Could you check a few things on this drawing? It's one solid part, dimensions in mm from its lowest x, y, z. A direction names the side the tool comes from. Give positions to 0.01 mm unless a question says otherwise; leave off trailing zeros. Loops run counter-clockwise (first coordinate to the right, second up) from the corner with the lowest first, then second, coordinate; pieces in that order, holes last. Notation, with made-up numbers: M 72.25,55 L 97.25,55 A19 ccw 97.25,88 Z; hole C 48.5,81.5 d8. An arc over 180 degrees is marked long. Answer as CSV lines item,"result". Start each with the question number.
Item 1: Will these pins go through, and if not, where does the flat tip stop? P1, Ø12, axis at x = 9.5, z = 9, coming from the -Y side; P2, Ø4, axis at x = 17.5, z = 22, coming from the +Y side; P3, Ø1.5, axis at x = 4, y = 7, coming from the -Z side; P4, Ø4, axis at x = 2.5, z = 23.5, coming from the +Y side.
Item 2: I want a section at D-D on y = 2.5. List the corners of the cut face in (x, z) for me, plus the area to 3 significant figures.
Item 3: I want a section at A-A on z = 14. List the corners of the cut face in (x, y) for me.
Item 4: I want a section at B-B on x = 11.25. List the corners of the cut face in (y, z) for me.
Item 5: If we mould it in two halves opening along Y, with no side actions, what happens to the marked faces 3, 4 and 5? For each: released by +Y, released by -Y, zero draft, split by the parting line, or undercut.
Item 6: For the marked faces 1 and 2, which set-ups out of +Z, -Z, +X, -X, +Y, -Y let a thin tool reach every point of the face, with its end or its side?
Item 7: I want a section at C-C on y = 12.25. List the corners of the cut face in (x, z) for me.
Item 8: If I drill on line 1 along X through (y, z) = (10, 27.25); line 2 along Z through (x, y) = (10, 3.95), over which ranges is the centre line in solid material (lowest first)? Write a range as from..to.
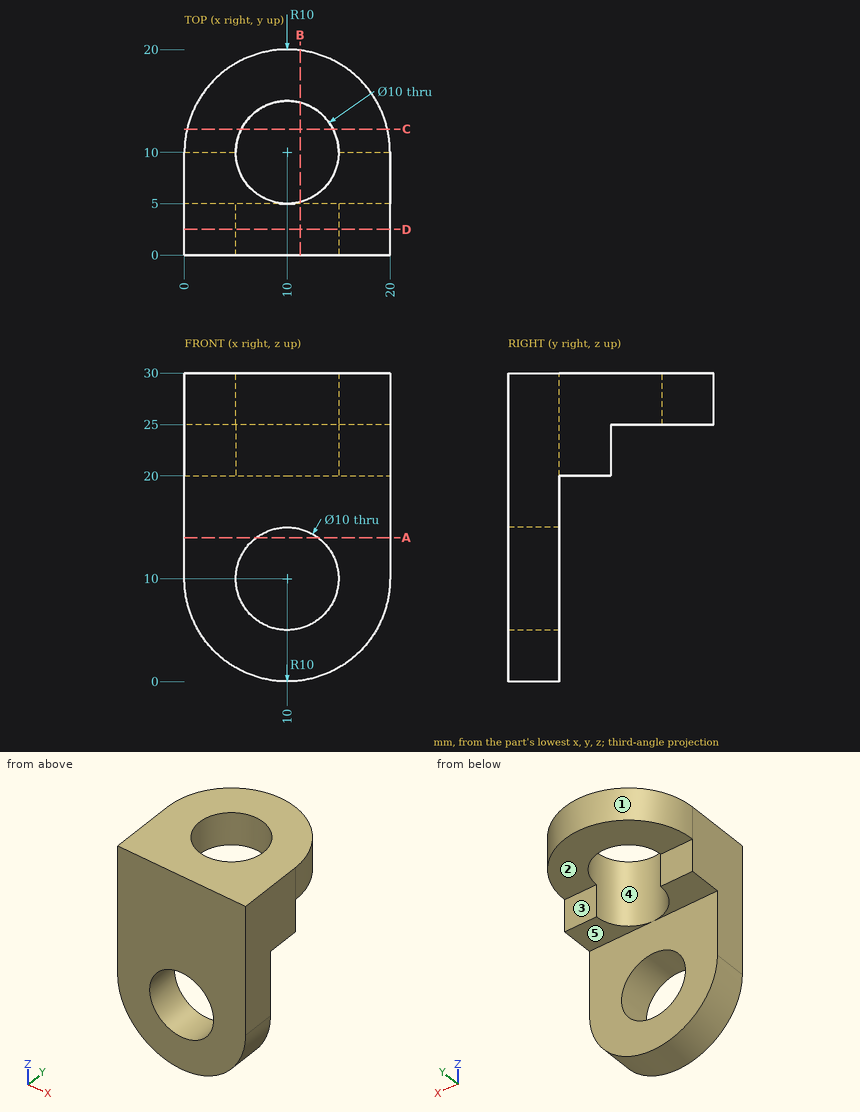
Result:
1,P1,"y = 0"
1,P2,"y = 10"
1,P3,"z = 20"
1,P4,"y = 17.86"
2,outline,"M 0,10 A10 ccw 20,10 L 20,30 L 0,30 Z; hole C 10,10 d10"
2,area,"479 mm^2"
3,outline,"M 0,0 L 7,0 L 7,5 L 0,5 Z; M 13,0 L 20,0 L 20,5 L 13,5 Z"
4,outline,"M 0,0.08 L 5,0.08 L 5,5.16 L 0,5.16 Z; M 0,14.84 L 5,14.84 L 5,20 L 5.16,20 L 5.16,30 L 0,30 Z; M 14.84,25 L 19.92,25 L 19.92,30 L 14.84,30 Z"
5,face 3,"released by +Y"
5,face 4,"undercut"
5,face 5,"zero draft"
6,face 1,"+Z, -Z, +Y"
6,face 2,"-Z, +X, -X, +Y"
7,outline,"M 0.26,25 L 5.53,25 L 5.53,30 L 0.26,30 Z; M 14.47,25 L 19.74,25 L 19.74,30 L 14.47,30 Z"
8,line 1,"0..5, 15..20"
8,line 2,"0..5, 15..30"
